from build123d import *

# Parameters (mm, degrees)
F0_R          = 28.2124188792
F1_DEPTH      = 25.4
F1_DEPTH_BACK = 25.4
F3_DEPTH      = 67.69626
F3_DEPTH_BACK = 44.95286


with BuildPart() as f1:
    # F0 (on Top) → F1 (new body, two sides)
    with BuildSketch(Plane.XY) as f1_sk:
        with BuildLine():
            ThreePointArc((115.9656523028, -15.875), (112.6573614726, 0), (115.9656523028, 15.875))
            Line((115.9656523028, 15.875), (-152.4, 15.875))
            Line((-152.4, 15.875), (-152.4, -15.875))
            Line((-152.4, -15.875), (115.9656523028, -15.875))
        make_face()
        with BuildLine():
            ThreePointArc((192.1426385274, 0), (160.5080270907, 38.906775937), (115.9656523028, 15.875))
            ThreePointArc((115.9656523028, 15.875), (112.6573614726, 0), (115.9656523028, -15.875))
            ThreePointArc((115.9656523028, -15.875), (160.5080270907, -38.906775937), (192.1426385274, 0))
        make_face()
        with Locations((152.4, 0)):
            Circle(F0_R, mode=Mode.SUBTRACT)
    extrude(amount=F1_DEPTH)
    extrude(f1_sk.sketch, amount=-F1_DEPTH_BACK)

    # F2 (on Front) → F3 (cut, two sides)
    with BuildSketch(Plane.XZ) as f3_sk:
        Polygon((72.0261707902, -3.3403777052), (-164.0271991491, 0), (-162.436529994, -48.5150068998), (115.6101450324, -51.6963265836), (115.6101450324, -25.9276945144), align=None)
    extrude(amount=-F3_DEPTH, mode=Mode.SUBTRACT)
    extrude(f3_sk.sketch, amount=F3_DEPTH_BACK, mode=Mode.SUBTRACT)

    # F4: F1 across face


with BuildPart() as f1_1:
    add(f1.part)
    add(f1.part.mirror(Plane(origin=(-152.4, 0, 12.6177320857), x_dir=(0, -1, 0), z_dir=(-1, 0, 0))))


solid = f1_1.part
Design review of the part built by this model. Coordinates are the model's own, in mm. A direction names the side the tool comes from. Round coordinates to 2 decimals unless told otherwise and drop trailing zeros. Write each loop counter-clockwise with the first axis right and the second up, starting at its lowest first coordinate (ties: lowest second). Pieces come first, ordered by that corner, then holes.
Item 1: For pin 1 Ø12.5 at (x, z) = (-17, -11.5) entering from -Y; pin 2 Ø1 at (x, z) = (103, -19) entering from +Y (3 decimals); pin 3 Ø10 at (y, z) = (21, -19) entering from -X; pin 4 Ø6 at (y, z) = (-6.5, 8) entering from +X, all flat-tipped, find the tip position at first contact; note any pin that passes through.
Item 2: Consider section B-B on x = 152.4. Give the boundary of the cut face in (y, z).
Item 3: Consider section D-D on x = -454.5. Give the boundary of the cut face in (y, z), and give its area (3 significant figures).
Item 4: For faces 1 (the flat face through (161.4, 27.1, -25.4)), 2 (the flat face through (-156, 15.875, 12)), list the 3-axis set-ups (+Z, -Z, +X, -X, +Y, -Y) from which the entire face can be reached by the end or side of a thin tool; tool diameter is ignored.
Item 5: Wall thickness on L1, parallel to Y at x = 154, z = -10; L2, parallel to X at y = 4.5, z = -11.5; L3, parallel to X at y = -22, z = 5.5: over which ranges is each line inside the solid? List them lowest first.
Item 6: Consider section C-C on z = 17. Give the boundary of the cut face in (x, y) (3 decimals).
Item 7: Consider section A-A on z = -15. Give the boundary of the cut face in (x, y) (3 decimals), and give its area (3 significant figures).
Check values:
1. pin 1: passes through
1. pin 2: stops at y = 15.875
1. pin 3: stops at x = -493.58
1. pin 4: stops at x = 191.99
2. outline: (-39.74, -25.4) - (-28.21, -25.4) - (-28.21, 25.4) - (-39.74, 25.4) - close; (28.21, -25.4) - (39.74, -25.4) - (39.74, 25.4) - (28.21, 25.4) - close
3. outline: (-39.65, -25.4) - (-28.08, -25.4) - (-28.08, 25.4) - (-39.65, 25.4) - close; (28.08, -25.4) - (39.65, -25.4) - (39.65, 25.4) - (28.08, 25.4) - close
3. area: 1,180 mm2
4. face 1: -Z, +X, -X, +Y, -Y
4. face 2: +Z, -Z, +Y
5. L1: y = -39.71 to -28.17, 28.17 to 39.71
5. L2: x = -496.69 to -485.05, -429.35 to -392.57, 87.77 to 124.55, 180.25 to 191.89
5. L3: x = -490.3 to -474.86, -439.54 to -424.1, 119.3 to 134.74, 170.06 to 185.5
6. outline: (-420.766, -15.875) - (115.966, -15.875) arc R39.743 ccw (long way) to (115.966, 15.875) - (-420.766, 15.875) arc R39.743 ccw (long way) to start; hole circle Ø56.425 at (-457.2, 0); hole circle Ø56.425 at (152.4, 0)
7. outline: (-420.766, -15.875) - (-399.324, -15.875) - (-399.324, 15.875) - (-420.766, 15.875) arc R39.743 ccw (long way) to start; (94.524, -15.875) - (115.966, -15.875) arc R39.743 ccw (long way) to (115.966, 15.875) - (94.524, 15.875) - close; hole circle Ø56.425 at (-457.2, 0); hole circle Ø56.425 at (152.4, 0)
7. area: 6,140 mm2
